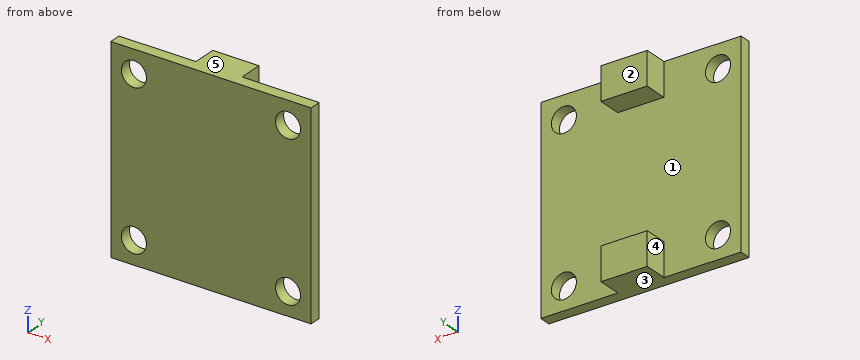
from build123d import *

# Parameters (mm, degrees)
SKETCH1_W           = 26
SKETCH1_H           = 26
BOSS_EXTRUDE1_DEPTH = 1.5
SKETCH2_R           = 1.625
CUT_EXTRUDE1_DEPTH  = 19.445866746
SKETCH3_W           = 6
SKETCH3_H           = 4.3
BOSS_EXTRUDE2_DEPTH = 3.1


with BuildPart() as part:
    # Sketch1 → Boss-Extrude1 (new body)
    with BuildSketch(Plane(origin=(0, 0, 0), x_dir=(1, 0, 0), z_dir=(0, 1, 0))):
        Rectangle(SKETCH1_W, SKETCH1_H)
    extrude(amount=BOSS_EXTRUDE1_DEPTH)

    # Sketch2 → Cut-Extrude1 (cut, through all)
    with BuildSketch(Plane(origin=(0, 1.5, 0), x_dir=(1, 0, 0), z_dir=(0, 1, 0))):
        with Locations(Location((-10, 10, 0), (0, 0, 270))):
            Circle(SKETCH2_R)
        with Locations(Location((10, 10, 0), (0, 0, 270))):
            Circle(SKETCH2_R)
        with Locations(Location((10, -10, 0), (0, 0, 270))):
            Circle(SKETCH2_R)
        with Locations(Location((-10, -10, 0), (0, 0, 270))):
            Circle(SKETCH2_R)
    extrude(amount=-CUT_EXTRUDE1_DEPTH, mode=Mode.SUBTRACT)

    # Sketch3 → Boss-Extrude2 (add)
    with BuildSketch(Plane(origin=(0, 1.5, 0), x_dir=(1, 0, 0), z_dir=(0, 1, 0))):
        with Locations((0, 10.85)):
            Rectangle(SKETCH3_W, SKETCH3_H)
        with Locations((0, -10.85)):
            Rectangle(SKETCH3_W, SKETCH3_H)
    extrude(amount=BOSS_EXTRUDE2_DEPTH)


solid = part.part
The model under review builds one solid part; all positions refer to its coordinate system, in mm. Face numbers are marked on the shaded views. A direction names the side the tool comes from. Round coordinates to 2 decimals unless told otherwise and drop trailing zeros. Write each loop counter-clockwise with the first axis right and the second up, starting at its lowest first coordinate (ties: lowest second). Pieces come first, ordered by that corner, then holes. Notation, with made-up numbers: (1.25, 43) - (29.25, 43) arc R24 cw to (29.25, 69) - close; hole circle Ø4 at (-7, 4.25). An arc over 180 degrees is marked (long way). One line per item, written item: value. Start each with the question number.
1. The part is to be moulded in two halves that separate along Z. For the marked faces 1, 2 and 3, say which applies: released by +Z, released by -Z, zero draft, split by the parting line, or undercut.
2. Consider section D-D on x = 2. Write out the cut boundary in (y, z), and give its area (3 significant figures).
3. To check wall thickness, follow L1, parallel to X at y = 0.5, z = 10 (3 decimals); L2, parallel to Z at x = -2.25, y = 2.1; L3, parallel to Y at x = 11.25, z = -1. State the ranges of each line that lie inside material, in increasing order. Write a range as from..to.
4. Machinability: for the marked faces 4 and 5, which of the approach directions +Z, -Z, +X, -X, +Y, -Y give a long, thin tool a straight path to every point of the face, cutting with its end or side? Answer none if there is none.
5. Consider section B-B on x = 10. Write out the cut boundary in (y, z) (3 decimals).
6. Consider section A-A on z = -10. Write out the cut boundary in (x, y) (3 decimals).
7. Clearance check with flat-ended pins moving along their axes: P1, Ø2.5, axis at y = 3.5, z = 10, coming from the +X side; P2, Ø4, axis at x = -10, z = -10, coming from the +Y side; P3, Ø2.5, axis at y = 4, z = -11.5, coming from the -X side. State where each tip first meets the part, or that it passes through.
8. Consider section C-C on y = 2.5. Write out the cut boundary in (x, z).
Checks:
1. face 1: undercut
1. face 2: zero draft
1. face 3: released by -Z
2. outline: (0, -13) - (4.6, -13) - (4.6, -8.7) - (1.5, -8.7) - (1.5, 8.7) - (4.6, 8.7) - (4.6, 13) - (0, 13) - close
2. area: 65.7 mm^2
3. L1: x = -13..-11.625, -8.375..8.375, 11.625..13
3. L2: z = -13..-8.7, 8.7..13
3. L3: y = 0..1.5
4. face 4: +Z, -Z, -X, +Y
4. face 5: +Z, +X, -X, +Y, -Y
5. outline: (0, -13) - (1.5, -13) - (1.5, -11.625) - (0, -11.625) - close; (0, -8.375) - (1.5, -8.375) - (1.5, 8.375) - (0, 8.375) - close; (0, 11.625) - (1.5, 11.625) - (1.5, 13) - (0, 13) - close
6. outline: (-13, 0) - (-11.625, 0) - (-11.625, 1.5) - (-13, 1.5) - close; (-8.375, 0) - (8.375, 0) - (8.375, 1.5) - (3, 1.5) - (3, 4.6) - (-3, 4.6) - (-3, 1.5) - (-8.375, 1.5) - close; (11.625, 0) - (13, 0) - (13, 1.5) - (11.625, 1.5) - close
7. P1: stops at x = 3
7. P2: stops at y = 1.5
7. P3: stops at x = -3
8. outline: (-3, -13) - (3, -13) - (3, -8.7) - (-3, -8.7) - close; (-3, 8.7) - (3, 8.7) - (3, 13) - (-3, 13) - close
